from build123d import *

# Parameters (mm, degrees)
PAD033_DEPTH            = 3
SKETCH041_R             = 4.6
PAD032_DEPTH            = 10
PAD035_DEPTH            = 16
PAD036_DEPTH            = 10
BODY010_PLACEMENT_ANGLE = 45


with BuildPart() as part:
    # Sketch042 → Pad033 (new body)
    with BuildSketch(Plane.XY):
        with BuildLine():
            Line((165, 21.235047), (53.12592, 21.235047))
            ThreePointArc((53.12592, 21.235047), (50.610162, 20.767349), (48.43058, 19.42675))
            ThreePointArc((48.43058, 19.42675), (39.806811, 0), (48.43058, -19.42675))
            ThreePointArc((48.43058, -19.42675), (50.610162, -20.767349), (53.12592, -21.235047))
            Line((53.12592, -21.235047), (165, -21.235047))
            ThreePointArc((165, -21.235047), (168.535534, -19.770581), (170, -16.235047))
            Line((170, -16.235047), (170, 16.235047))
            ThreePointArc((170, 16.235047), (168.535534, 19.770581), (165, 21.235047))
        make_face()
    extrude(amount=-PAD033_DEPTH)

    # Sketch041 → Pad032 (join)
    with BuildSketch(Plane.XY):
        with Locations((53.12592, 14.235047)):
            Circle(SKETCH041_R)
        with Locations((53.12592, -14.235047)):
            Circle(SKETCH041_R)
    extrude(amount=PAD032_DEPTH)

    # Sketch045 → Pad035 (join, symmetric)
    with BuildSketch(Plane.XZ):
        with BuildLine():
            Line((170, 0), (170, 15))
            Line((170, 15), (167, 15))
            ThreePointArc((152, 0), (162.606602, 4.393398), (167, 15))
            Line((152, 0), (170, 0))
        make_face()
    extrude(amount=PAD035_DEPTH, both=True)

    # Sketch046 → Pad036 (join)
    with BuildSketch(Plane.XY):
        with BuildLine():
            ThreePointArc((55.057772, 14.752686), (52.608282, 16.166899), (51.194069, 13.717409))
            ThreePointArc((51.194069, -13.717409), (53, 0), (51.194069, 13.717409))
            ThreePointArc((51.194069, -13.717409), (52.608281, -16.166899), (55.057771, -14.752689))
            ThreePointArc((55.057771, -14.752689), (57, -2e-06), (55.057772, 14.752686))
        make_face()
    extrude(amount=PAD036_DEPTH)


with BuildPart() as part_1:
    # Body010 placement: moved
    add(part.part.moved(Location((0, 0, -245))).rotate(Axis((0, 0, -245), (0, 0, 1)), BODY010_PLACEMENT_ANGLE))


solid = part_1.part
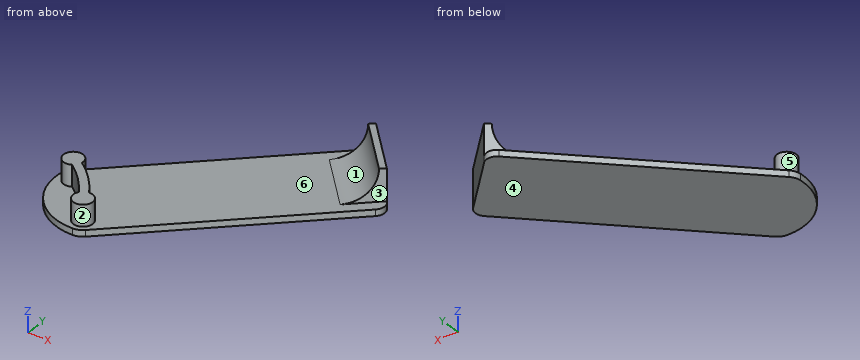
Read the model definition and answer for the solid it produces. Units are mm, in the model's axes. Face numbers are marked on the shaded views. A direction names the side the tool comes from. Give positions to 0.01 mm unless a question says otherwise; leave off trailing zeros. Loops run counter-clockwise (first coordinate to the right, second up) from the corner with the lowest first, then second, coordinate; pieces in that order, holes last. Notation, with made-up numbers: (24.25, 29) -> (69.25, 29) arc R15 ccw to (69.25, 48) -> close; hole circle Ø2 at (60, -1). An arc over 180 degrees is marked (long way). Answer as CSV lines item,"result".
Item 1: Determine the mould class of the marked faces 4, 5 and 6 for opening direction Z: +Z half, -Z half, draft (parallel to the pull), parting line (faces both ways), or undercut.
Returned:
face 4,"-Z half"
face 5,"draft"
face 6,"+Z half"
Item 2: Find section B-B on x = 27.5. Give the vertices of the cut face in (y, z).
Returned:
outline,"(28.82, -248) -> (57.53, -248) -> (57.53, -245) -> (52.23, -245) -> (52.23, -235) -> (43.03, -235) -> (43.03, -245) -> (28.82, -245) -> close"
Item 3: For the marked faces 1, 2 and 3, determine the directions among +Z, -Z, +X, -X, +Y, -Y from which every point of the face is accessible in a straight line to the end or side of a thin tool.
Returned:
face 1,"+Z, -X, -Y"
face 2,"+Z"
face 3,"+Z, +X, -Y"
Item 4: Find section C-C on y = 35.5. Give the vertices of the cut face in (x, z).
Returned:
outline,"(22.98, -248) -> (65.53, -248) -> (65.53, -245) -> (44.6, -245) -> (44.6, -235) -> (39.35, -235) -> (39.35, -245) -> (22.98, -245) -> close"
Item 5: Each of these flat-tipped pins is pushed along its axis until it touches: pin 1 (5 mm diameter, centred on x = 63.5, z = -244, fed in from +Y); pin 2 (5 mm diameter, centred on y = 105.5, z = -236, fed in from +X); pin 3 (9 mm diameter, centred on x = 43.5, y = 39, fed in from +Z). Where does it stop, or does it pass through?
Returned:
pin 1,"stops at y = 95.82"
pin 2,"stops at x = 130.63"
pin 3,"stops at z = -235"
Item 6: Find section A-A on z = -241.25. Give the vertices of the cut face in (x, y), plus the area to 3 significant figures.
Returned:
outline,"(29.94, 43.73) arc R53 cw to (43.73, 29.94) arc R4.6 ccw (long way) to (47.12, 32.07) arc R57 ccw to (32.07, 47.12) arc R4.6 ccw (long way) to start; (103.18, 125.81) -> (125.81, 103.18) -> (131.52, 108.89) -> (108.89, 131.52) -> close"
area,"471 mm²"
Item 7: Consider line 1 (Z direction, x = 80, y = 82.5); line 2 (X direction, y = 117.5, z = -247); line 3 (Y direction, x = 49.5, z = -240.5). Determine where each line is inside the solid, lowest interval first. Write a range as [from, to].
Returned:
line 1,"z = [-248, -245]"
line 2,"x = [87.47, 122.92]"
line 3,"y = [23.3, 31.7]"
Item 8: Find section D-D on z = -233.5. Give the vertices of the cut face in (x, y).
Returned:
outline,"(106.48, 129.11) -> (129.11, 106.48) -> (131.52, 108.89) -> (108.89, 131.52) -> close"
